For this review, take the finished solid that the model builds, in its own axes (mm). Round coordinates to 2 decimals unless told otherwise and drop trailing zeros. Order: outer loops, then holes, each group sorted by start corner. A loop starts at its lowest first (then second) coordinate and runs counter-clockwise, first axis right, second up. Notation, with made-up numbers: (23, -7) - (38, -7) arc R15 cw to (38, 0) - close; hole circle Ø2 at (47, -15). An arc over 180 degrees is marked (long way). One line per question, with ' | ' between items.
```python
from build123d import *

# Parameters (mm, degrees)
SKETCH_F_W                   = 449
SKETCH_F_H                   = 79
SKETCH_F_R                   = 3.25
ESTRUSIONE_ESTRUSIONE1_DEPTH = 5
SKETCH1_R                    = 1.75
EXTRUDE1_DEPTH               = 6


with BuildPart() as part:
    # Sketch f → Estrusione-Estrusione1 (new body)
    with BuildSketch(Plane.XY):
        with Locations((224.5, 39.5)):
            Rectangle(SKETCH_F_W, SKETCH_F_H)
        with Locations((11.5, 67.5)):
            Circle(SKETCH_F_R, mode=Mode.SUBTRACT)
        with Locations((437.5, 67.5)):
            Circle(SKETCH_F_R, mode=Mode.SUBTRACT)
        with Locations((11.5, 11.5)):
            Circle(SKETCH_F_R, mode=Mode.SUBTRACT)
        with Locations((437.5, 11.5)):
            Circle(SKETCH_F_R, mode=Mode.SUBTRACT)
    extrude(amount=ESTRUSIONE_ESTRUSIONE1_DEPTH)

    # Sketch1 → Extrude1 (cut, through all)
    with BuildSketch(Plane(origin=(0, 0, 0), x_dir=(-1, 0, 0), z_dir=(0, 0, -1))):
        with Locations((-341.3246338, 39.505506417)):
            Circle(SKETCH1_R)
        with Locations((-413.8246338, 39.505506417)):
            Circle(SKETCH1_R)
        with BuildLine():
            Line((-349.0746338, 55.5), (-406.0746338, 55.5))
            ThreePointArc((-406.0746338, 55.5), (-408.903060925, 54.328427125), (-410.0746338, 51.5))
            Line((-410.0746338, 51.5), (-410.0746338, 27.5))
            ThreePointArc((-410.0746338, 27.5), (-408.903060925, 24.671572875), (-406.0746338, 23.5))
            Line((-406.0746338, 23.5), (-349.0746338, 23.5))
            ThreePointArc((-349.0746338, 23.5), (-346.246206675, 24.671572875), (-345.0746338, 27.5))
            Line((-345.0746338, 27.5), (-345.0746338, 51.5))
            ThreePointArc((-345.0746338, 51.5), (-346.246206675, 54.328427125), (-349.0746338, 55.5))
        make_face()
    extrude(amount=-EXTRUDE1_DEPTH, mode=Mode.SUBTRACT)


solid = part.part
```
(1) For probe 1 along X at (y, z) = (39, 1.85); probe 2 along Y at (x, z) = (11.5, 1.65); probe 3 along X at (y, z) = (29.5, 4.15), list the stretches that pass through material, from the lowest coordinate up. Write a range as [from, to].
Output values:
probe 1: [0, 339.65], [343, 345.07], [410.07, 412.15], [415.5, 449] | probe 2: [0, 8.25], [14.75, 64.25], [70.75, 79] | probe 3: [0, 345.07], [410.07, 449]
(2) We need section A-A on x = 354.5. State the section outline as (y, z) points, plus the area to 3 significant figures.
Output values:
outline: (0, 0) - (23.5, 0) - (23.5, 5) - (0, 5) - close; (55.5, 0) - (79, 0) - (79, 5) - (55.5, 5) - close | area: 235 mm^2
(3) We need section B-B on y = 45.5. State the section outline as (x, z) points.
Output values:
outline: (0, 0) - (345.07, 0) - (345.07, 5) - (0, 5) - close; (410.07, 0) - (449, 0) - (449, 5) - (410.07, 5) - close
(4) We need section C-C on z = 1. State the section outline as (x, y) points, plus the area to 3 significant figures.
Output values:
outline: (0, 0) - (449, 0) - (449, 79) - (0, 79) - close; hole circle Ø6.5 at (11.5, 11.5); hole circle Ø6.5 at (11.5, 67.5); hole circle Ø3.5 at (341.32, 39.51); hole (345.07, 27.5) arc R4 ccw to (349.07, 23.5) - (406.07, 23.5) arc R4 ccw to (410.07, 27.5) - (410.07, 51.5) arc R4 ccw to (406.07, 55.5) - (349.07, 55.5) arc R4 ccw to (345.07, 51.5) - close; hole circle Ø3.5 at (413.82, 39.51); hole circle Ø6.5 at (437.5, 11.5); hole circle Ø6.5 at (437.5, 67.5) | area: 33,300 mm^2
